from build123d import *

# Parameters (mm, degrees)
SKETCH2_R           = 11.4554
BOSS_EXTRUDE1_DEPTH = 19.05
SKETCH3_R           = 5.08
CUT_EXTRUDE1_DEPTH  = 12.7


with BuildPart() as part:
    # Sketch1 → Revolve1 (revolve)
    with BuildSketch(Plane.XY, mode=Mode.PRIVATE) as revolve1_sk:
        Polygon((0, 19.05), (0, 0), (30.099, 18.085303772), (30.099, 19.355303772), (29.21, 19.355303772), (29.21, 21.260303772), (30.099, 21.260303772), (30.099, 27.610303772), (29.21, 27.610303772), (29.21, 29.515303772), (30.099, 29.515303772), (30.099, 30.785303772), (0, 30.785303772), align=None)
    revolve(revolve1_sk.sketch.rotate(Axis((0, 30.785303772, 0), (0, -1, 0)), 180), axis=Axis((0, 30.785303772, 0), (0, -1, 0)))

    # Sketch2 → Boss-Extrude1 (add)
    with BuildSketch(Plane(origin=(0, 30.785303772, 0), x_dir=(1, 0, 0), z_dir=(0, 1, 0))):
        Circle(SKETCH2_R)
    extrude(amount=BOSS_EXTRUDE1_DEPTH)

    # Sketch3 → Cut-Extrude1 (cut)
    with BuildSketch(Plane(origin=(0, 49.835303772, 0), x_dir=(1, 0, 0), z_dir=(0, 1, 0))):
        with Locations(Location((0, 0, 0), (0, 0, 180))):
            Circle(SKETCH3_R)
    extrude(amount=-CUT_EXTRUDE1_DEPTH, mode=Mode.SUBTRACT)


solid = part.part
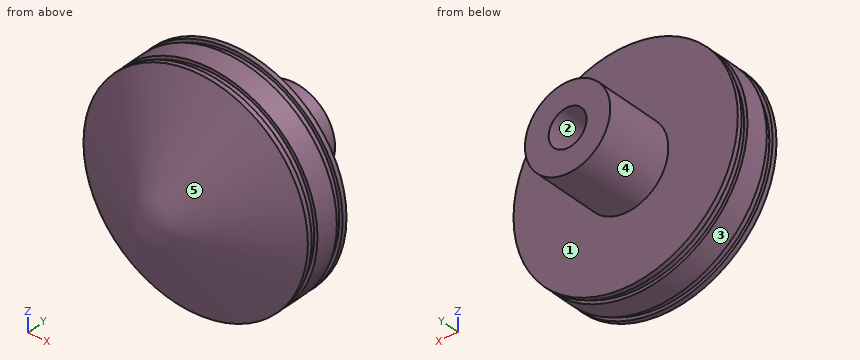
Geometry: final body of the model. Coordinates: model frame, mm. Face numbers are marked on the shaded views. A direction names the side the tool comes from. Give positions to 0.01 mm unless a question says otherwise; leave off trailing zeros. Write each loop counter-clockwise with the first axis right and the second up, starting at its lowest first coordinate (ties: lowest second). Pieces come first, ordered by that corner, then holes. Notation, with made-up numbers: (41.5, -30) -> (89.5, -30) arc R25 cw to (89.5, -15) -> close; hole circle Ø5 at (74, 45). An arc over 180 degrees is marked (long way). Answer as a JSON object with one key per item and string values.
1. Cut plane B-B on y = 24.5. Output: boundary loops of the cut face in (x, z), and give its area (3 significant figures).
Ans:
{"outline": "circle Ø60.2 at (0, 0)", "area": "2,850 mm^2"}
2. Cut plane C-C on y = 12. Output: boundary loops of the cut face in (x, z).
Ans:
{"outline": "circle Ø39.94 at (0, 0)"}
3. Contact query for flat-ended pins moving along their axis: pin 1 (5 mm diameter, centred on x = -12.5, z = 11, fed in from -Y); pin 2 (1 mm diameter, centred on x = -12, z = 19, fed in from -Y); pin 3 (8 mm diameter, centred on x = 16.5, z = -3.5, fed in from -Y). Output: stop coordinate, or through.
Ans:
{"pin 1": "stops at y = 8.5", "pin 2": "stops at y = 13.2", "pin 3": "stops at y = 7.73"}
4. Access query for the marked faces 4 and 5. Directions: +Z, -Z, +X, -X, +Y, -Y. A direction counts if a zero-diameter tool reaches every point of the face in a straight line with its end or side. Return the directions, or none.
Ans:
{"face 4": "+Y", "face 5": "-Y"}
5. Mould query, pull axis Z, two halves, no side actions, for the marked faces 1, 2 and 3. Classes: pulls with the +Z half, pulls with the -Z half, needs draft (parallel to the pull), parting line crosses it, or undercut.
Ans:
{"face 1": "needs draft", "face 2": "undercut", "face 3": "parting line crosses it"}
6. Cut plane A-A on y = 39. Output: boundary loops of the cut face in (x, z), and give its area (3 significant figures).
Ans:
{"outline": "circle Ø22.91 at (0, 0); hole circle Ø10.16 at (0, 0)", "area": "331 mm^2"}
7. Ray query, probe 1 along Z at (x, y) = (0, 42.75); probe 2 along Y at (x, z) = (-17.5, 16.5); probe 3 along Y at (x, z) = (-23.5, 10.5). Return the intervals inside material, ascending. Write a range as from..to.
Ans:
{"probe 1": "z = -11.46..-5.08, 5.08..11.46", "probe 2": "y = 14.45..30.79", "probe 3": "y = 15.47..30.79"}
